Read the model definition and answer for the solid it produces. Units are mm, in the model's axes. A direction names the side the tool comes from. Coordinates: 2 decimals unless noted, no trailing zeros. Order: outer loops, then holes, each group sorted by start corner. A loop starts at its lowest first (then second) coordinate and runs counter-clockwise, first axis right, second up. Notation, with made-up numbers: (18.5, -24.75) -> (46.5, -24.75) arc R17 ccw to (46.5, 0.25) -> close; hole circle Ø7 at (-7, 43.5). An arc over 180 degrees is marked (long way). Answer as a JSON object with one key per item and string values. Group by question number.
1) Determine the mould class of faces 1 (the cylindrical face through (103.67, -19.961, -10.382)), 2 (the flat face through (10, 4.6, 22.4)), 3 (the cylindrical face through (2.99, -31.52, -0.33)), 4 (the flat face through (1, 5.7, 30.5)) for opening direction Y: released by +Y, released by -Y, zero draft, split by the parting line, or undercut.
2) Section C-C on y = -16 is taken. Determine the outline of the cut face in (x, z), and give its area (3 significant figures).
3) Consider L1, parallel to Y at x = 133, z = 0.5; L2, parallel to X at y = -16, z = -18; L3, parallel to Y at x = 25.5, z = -13.5. Determine where each line is inside the solid, lowest interval first.
4) Section B-B on z = -26 is taken. Determine the outline of the cut face in (x, y).
5) A tool of negligible diameter and unlimited length cuts with its end or side. For faces 5 (the cylindrical face through (0.493, -0.772, 37.492)), 6 (the cylindrical face through (5, 0, -29)), from which of +Z, -Z, +X, -X, +Y, -Y can it reach the whole face along a straight path? Write none if from no direction.
6) Given pin 1 (10 mm diameter, centred on x = 144.5, y = 5.5, fed in from -Z); pin 2 (2 mm diameter, centred on y = 15, z = -34, fed in from +X); pin 3 (2.5 mm diameter, centred on y = 34, z = 1, fed in from -X), each flat-ended and moving along its own axis, determine where each tip first touches the part or whether it passes through.
7) Section A-A on y = 0 is taken. Count the separate pieces of the cut face and the enclosed holes in it, and give its area (3 significant figures).
from build123d import *

# Parameters (mm, degrees)
SKETCH2_R               = 55
BOSS_EXTRUDE1_DEPTH     = 10
SKETCH3_R               = 22.5
BOSS_EXTRUDE2_DEPTH     = 190
SKETCH4_R               = 19
CUT_EXTRUDE1_DEPTH      = 1
CUT_EXTRUDE1_DEPTH_BACK = 201
SKETCH14_R              = 37.5
SKETCH14_R_2            = 30.5
CUT_EXTRUDE5_DEPTH      = 1
SKETCH15_R              = 38
SKETCH15_R_2            = 30
CUT_EXTRUDE6_DEPTH      = 4
SKETCH16_R              = 2.5
CUT_EXTRUDE7_DEPTH      = 4
SKETCH17_R              = 5
CUT_EXTRUDE8_DEPTH      = 2
SKETCH20_R              = 3
CUT_EXTRUDE9_DEPTH      = 10
SKETCH21_R              = 3
CUT_EXTRUDE10_DEPTH     = 10


with BuildPart() as part:
    # Sketch2 → Boss-Extrude1 (new body)
    with BuildSketch(Plane(origin=(0, 0, 0), x_dir=(0, 0, -1), z_dir=(1, 0, 0))):
        Circle(SKETCH2_R)
    extrude(amount=BOSS_EXTRUDE1_DEPTH)

    # Sketch3 → Boss-Extrude2 (add)
    with BuildSketch(Plane(origin=(10, 0, 0), x_dir=(0, 0, -1), z_dir=(1, 0, 0))):
        Circle(SKETCH3_R)
    extrude(amount=BOSS_EXTRUDE2_DEPTH)

    # Sketch4 → Cut-Extrude1 (cut, two sides)
    with BuildSketch(Plane.ZY) as cut_extrude1_sk:
        Circle(SKETCH4_R)
    extrude(amount=CUT_EXTRUDE1_DEPTH, mode=Mode.SUBTRACT)
    extrude(cut_extrude1_sk.sketch, amount=-CUT_EXTRUDE1_DEPTH_BACK, mode=Mode.SUBTRACT)

    # Sketch14 → Cut-Extrude5 (cut)
    with BuildSketch(Plane.ZY):
        Circle(SKETCH14_R)
        Circle(SKETCH14_R_2, mode=Mode.SUBTRACT)
    extrude(amount=-CUT_EXTRUDE5_DEPTH, mode=Mode.SUBTRACT)

    # Sketch15 → Cut-Extrude6 (cut)
    with BuildSketch(Plane(origin=(10, 0, 0), x_dir=(0, 0, -1), z_dir=(1, 0, 0))):
        Circle(SKETCH15_R)
        Circle(SKETCH15_R_2, mode=Mode.SUBTRACT)
    extrude(amount=-CUT_EXTRUDE6_DEPTH, mode=Mode.SUBTRACT)

    # Sketch16 → Cut-Extrude7 (cut)
    with BuildSketch(Plane.ZY):
        with Locations((0, 34)):
            Circle(SKETCH16_R)
        with Locations((0, -34)):
            Circle(SKETCH16_R)
    extrude(amount=-CUT_EXTRUDE7_DEPTH, mode=Mode.SUBTRACT)

    # Sketch17 → Cut-Extrude8 (cut)
    with BuildSketch(Plane.ZY):
        with Locations((0, -34)):
            Circle(SKETCH17_R)
        with Locations((0, 34)):
            Circle(SKETCH17_R)
    extrude(amount=-CUT_EXTRUDE8_DEPTH, mode=Mode.SUBTRACT)

    # Sketch20 → Cut-Extrude9 (cut)
    with BuildSketch(Plane.ZY):
        with Locations((-26, 0)):
            Circle(SKETCH20_R)
    extrude(amount=-CUT_EXTRUDE9_DEPTH, mode=Mode.SUBTRACT)

    # Sketch21 → Cut-Extrude10 (cut)
    with BuildSketch(Plane.ZY):
        with Locations((0, 45)):
            Circle(SKETCH21_R)
    extrude(amount=-CUT_EXTRUDE10_DEPTH, mode=Mode.SUBTRACT)


solid = part.part
Worked answers:
{
 "1": {"face 1": "split by the parting line", "face 2": "zero draft", "face 3": "undercut", "face 4": "undercut"},
 "2": {"outline": "(0, -52.62) -> (10, -52.62) -> (10, -34.47) -> (6, -34.47) -> (6, -25.38) -> (10, -25.38) -> (10, -15.82) -> (200, -15.82) -> (200, -10.25) -> (0, -10.25) -> (0, -25.97) -> (1, -25.97) -> (1, -33.92) -> (0, -33.92) -> close; (0, 10.25) -> (200, 10.25) -> (200, 15.82) -> (10, 15.82) -> (10, 25.38) -> (6, 25.38) -> (6, 34.47) -> (10, 34.47) -> (10, 52.62) -> (0, 52.62) -> (0, 33.92) -> (1, 33.92) -> (1, 25.97) -> (0, 25.97) -> close", "area": "2,880 mm²"},
 "3": {"L1": "y = -22.49 to -18.99, 18.99 to 22.49", "L2": "x = 0 to 10", "L3": "y = -18 to -13.37, 13.37 to 18"},
 "4": {"outline": "(0, -48.47) -> (10, -48.47) -> (10, -27.71) -> (6, -27.71) -> (6, -14.97) -> (10, -14.97) -> (10, -3) -> (0, -3) -> (0, -15.95) -> (1, -15.95) -> (1, -27.02) -> (0, -27.02) -> close; (0, 3) -> (10, 3) -> (10, 14.97) -> (6, 14.97) -> (6, 27.71) -> (10, 27.71) -> (10, 48.47) -> (0, 48.47) -> (0, 27.02) -> (1, 27.02) -> (1, 15.95) -> (0, 15.95) -> close"},
 "5": {"face 5": "-X", "face 6": "+X, -X"},
 "6": {"pin 1": "stops at z = -22.49", "pin 2": "stops at x = 10", "pin 3": "stops at x = 4"},
 "7": {"separate pieces": "3", "enclosed holes": "0", "area": "1,910 mm²"}
}
